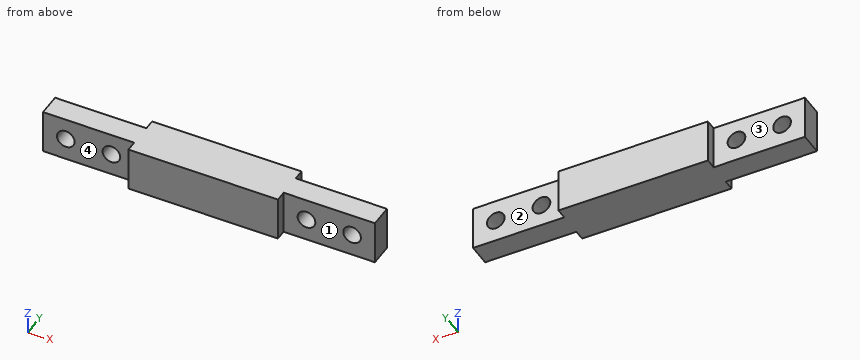
from build123d import *

# Parameters (mm, degrees)
PAD_DEPTH       = 7.8
SKETCH001_R     = 1.55
POCKET_DEPTH    = 5.901
POCKET001_DEPTH = 5.901


with BuildPart() as part:
    # Sketch → Pad (new body)
    with BuildSketch(Plane.XY):
        Polygon((29.1, -2), (29.1, 2), (13.1, 2), (13.1, 3.9), (-13.1, 3.9), (-13.1, 2), (-29.1, 2), (-29.1, -2), (-13.1, -2), (-13.1, -3.9), (13.1, -3.9), (13.1, -2), align=None)
    extrude(amount=PAD_DEPTH)

    # Sketch001 (on Face3 of Pad) → Pocket (cut, through all)
    with BuildSketch(Plane.XZ.offset(2)):
        with Locations((-25.1, 3.95)):
            Circle(SKETCH001_R)
        with Locations((-17.1, 3.95)):
            Circle(SKETCH001_R)
        with Locations((17.1, 3.95)):
            Circle(SKETCH001_R)
        with Locations((25.1, 3.95)):
            Circle(SKETCH001_R)
    extrude(amount=-POCKET_DEPTH, mode=Mode.SUBTRACT)

    # Sketch001 (on Face3 of Pad) → Pocket001 (cut, through all)
    with BuildSketch(Plane.XZ.offset(2)):
        with Locations((-25.1, 3.95)):
            Circle(SKETCH001_R)
        with Locations((-17.1, 3.95)):
            Circle(SKETCH001_R)
        with Locations((17.1, 3.95)):
            Circle(SKETCH001_R)
        with Locations((25.1, 3.95)):
            Circle(SKETCH001_R)
    extrude(amount=-POCKET001_DEPTH, mode=Mode.SUBTRACT)


solid = part.part
CAD build for the part. Positions are in the model's coordinates, mm. Face numbers are marked on the shaded views. A direction names the side the tool comes from. Coordinates: 2 decimals unless noted, no trailing zeros. Order: outer loops, then holes, each group sorted by start corner. A loop starts at its lowest first (then second) coordinate and runs counter-clockwise, first axis right, second up.
Item 1: Band-saw the part on A-A on x = -17.1. List the corners of the cut face in (y, z).
Check sheet entries:
outline: (-2, 0) - (2, 0) - (2, 2.4) - (-2, 2.4) - close; (-2, 5.5) - (2, 5.5) - (2, 7.8) - (-2, 7.8) - close
Item 2: Drill centre lines: L1, parallel to Z at x = 17.1, y = 1; L2, parallel to X at y = -0.25, z = 4.25; L3, parallel to X at y = 3.5, z = 3. Where is each one in solid material? Low to high.
Check sheet entries:
L1: z = 0 to 2.4, 5.5 to 7.8
L2: x = -29.1 to -26.62, -23.58 to -18.62, -15.58 to 15.58, 18.62 to 23.58, 26.62 to 29.1
L3: x = -13.1 to 13.1
Item 3: 3-axis set-ups, long thin cutter, end or side, ignore diameter. For the marked faces 1, 2, 3 and 4: which of +Z, -Z, +X, -X, +Y, -Y reach the whole face in a straight line?
Check sheet entries:
face 1: +Z, -Z, +X, -Y
face 2: +Z, -Z, +X, +Y
face 3: +Z, -Z, -X, +Y
face 4: +Z, -Z, -X, -Y
Item 4: Band-saw the part on D-D on x = 21. List the corners of the cut face in (y, z), plus the area to 3 significant figures.
Check sheet entries:
outline: (-2, 0) - (2, 0) - (2, 7.8) - (-2, 7.8) - close
area: 31.2 mm2
Item 5: Pin check, flat tips, straight feed: pin 1 Ø4 at (x, z) = (21, 4) entering from -Y; pin 2 Ø2.5 at (x, z) = (-18.5, 3.5) entering from +Y; pin 3 Ø1.9 at (x, z) = (25.1, 3.95) entering from +Y; pin 4 Ø0.6 at (y, z) = (-3.5, 2.5) entering from +X. Stop position of each tip, or through.
Check sheet entries:
pin 1: stops at y = -2
pin 2: stops at y = 2
pin 3: passes through
pin 4: stops at x = 13.1
Item 6: Band-saw the part on B-B on y = 1. List the corners of the cut face in (x, z), plus the area to 3 significant figures.
Check sheet entries:
outline: (-29.1, 0) - (29.1, 0) - (29.1, 7.8) - (-29.1, 7.8) - close; hole circle Ø3.1 at (-25.1, 3.95); hole circle Ø3.1 at (-17.1, 3.95); hole circle Ø3.1 at (17.1, 3.95); hole circle Ø3.1 at (25.1, 3.95)
area: 424 mm2
Item 7: Band-saw the part on C-C on z = 3.95. List the corners of the cut face in (x, y).
Check sheet entries:
outline: (-29.1, -2) - (-26.65, -2) - (-26.65, 2) - (-29.1, 2) - close; (-23.55, -2) - (-18.65, -2) - (-18.65, 2) - (-23.55, 2) - close; (-15.55, -2) - (-13.1, -2) - (-13.1, -3.9) - (13.1, -3.9) - (13.1, -2) - (15.55, -2) - (15.55, 2) - (13.1, 2) - (13.1, 3.9) - (-13.1, 3.9) - (-13.1, 2) - (-15.55, 2) - close; (18.65, -2) - (23.55, -2) - (23.55, 2) - (18.65, 2) - close; (26.65, -2) - (29.1, -2) - (29.1, 2) - (26.65, 2) - close
